Read the model definition and answer for the solid it produces. Units are mm, in the model's axes. A direction names the side the tool comes from. Give positions to 0.01 mm unless a question says otherwise; leave off trailing zeros. Order: outer loops, then holes, each group sorted by start corner. A loop starts at its lowest first (then second) coordinate and runs counter-clockwise, first axis right, second up. Notation, with made-up numbers: (-16.5, -30) -> (38.5, -30) arc R21 ccw to (38.5, -18) -> close; hole circle Ø10 at (9.5, 49.25). An arc over 180 degrees is marked (long way). Use one line per item in the form item = value.
```python
from build123d import *

# Parameters (mm, degrees)
SALIENTE_EXTRUIR1_DEPTH = 2
SALIENTE_EXTRUIR2_DEPTH = 24
CROQUIS4_W              = 26.838471133
CROQUIS4_H              = 14
CORTAR_EXTRUIR1_DEPTH   = 70.1
SALIENTE_EXTRUIR3_DEPTH = 2
SALIENTE_EXTRUIR4_DEPTH = 2
CROQUIS7_W              = 41.5
CROQUIS7_H              = 2
SALIENTE_EXTRUIR5_DEPTH = 8
SALIENTE_EXTRUIR6_DEPTH = 6


with BuildPart() as part:
    # Croquis1 → Saliente-Extruir1 (new body)
    with BuildSketch(Plane.XY):
        Polygon((-48.939551095, 26.503456625), (-8.439551095, 26.503456625), (-8.439551095, 6.503456625), (-8.439551095, 5.503456625), (-48.939551095, 5.503456625), (-49.939551095, 5.503456625), (-49.939551095, 26.503456625), align=None)
    extrude(amount=SALIENTE_EXTRUIR1_DEPTH)

    # Croquis3 → Saliente-Extruir2 (add)
    with BuildSketch(Plane.XY):
        Polygon((-48.939551095, 26.503456625), (-8.439551095, 26.503456625), (-8.439551095, 6.503456625), (-8.439551095, 5.503456625), (-48.939551095, 5.503456625), (-49.939551095, 5.503456625), (-49.939551095, 26.503456625), align=None)
        Polygon((-46.939551095, 7.503456625), (-47.939551095, 7.503456625), (-47.939551095, 24.503456625), (-46.939551095, 24.503456625), (-10.439551095, 24.503456625), (-10.439551095, 8.503456625), (-10.439551095, 7.503456625), align=None, mode=Mode.SUBTRACT)
    extrude(amount=SALIENTE_EXTRUIR2_DEPTH)

    # Croquis4 → Cortar-Extruir1 (cut)
    with BuildSketch(Plane(origin=(0, 0, 0), x_dir=(0, 0, -1), z_dir=(1, 0, 0))):
        with Locations((-15.419235567, 16.503456625)):
            Rectangle(CROQUIS4_W, CROQUIS4_H)
    extrude(amount=-CORTAR_EXTRUIR1_DEPTH, mode=Mode.SUBTRACT)

    # Croquis5 → Saliente-Extruir3 (add)
    with BuildSketch(Plane(origin=(0, 26.503456625, 0), x_dir=(1, 0, 0), z_dir=(0, 1, 0))):
        Polygon((-49.939551095, -20.607192887), (-8.439551095, -20.607192887), (-8.439551095, -24), (-8.439551095, -36.1), (-48.939551095, -36.1), (-49.939551095, -36.1), align=None)
    extrude(amount=-SALIENTE_EXTRUIR3_DEPTH)

    # Croquis6 → Saliente-Extruir4 (add)
    with BuildSketch(Plane.XY.offset(36.1)):
        Polygon((-8.439551095, 24.503456625), (-8.439551095, 33.503456625), (-48.939551095, 33.503456625), (-49.939551095, 33.503456625), (-49.939551095, 24.503456625), align=None)
    extrude(amount=-SALIENTE_EXTRUIR4_DEPTH)

    # Croquis7 → Saliente-Extruir5 (add)
    with BuildSketch(Plane.XY.offset(36.1)):
        with Locations((-29.189551095, 32.503456625)):
            Rectangle(CROQUIS7_W, CROQUIS7_H)
    extrude(amount=-SALIENTE_EXTRUIR5_DEPTH)

    # Croquis8 → Saliente-Extruir6 (add)
    with BuildSketch(Plane.XY.offset(36.1)):
        Polygon((-49.939551095, 29.503456625), (-49.939551095, 26.503456625), (-49.715027183, 26.503456625), (-8.439551095, 26.503456625), (-8.439551095, 29.503456625), (-49.715027183, 29.503456625), align=None)
    extrude(amount=-SALIENTE_EXTRUIR6_DEPTH)


solid = part.part
```
Item 1: The part is cut by section C-C on y = 27.25. Give the vertices of the cut face in (x, z).
Checks:
outline = (-49.94, 30.1) -> (-8.44, 30.1) -> (-8.44, 36.1) -> (-49.94, 36.1) -> close
Item 2: Which of the six approach directions +Z, -Z, +X, -X, +Y, -Y give full straight-line access (tool end or side, diameter ignored) to faces 1 (the flat face through (-10.44, 24, 13)), 2 (the flat face through (-49, 24, 24)), 3 (the flat face through (-49, 9.503, 13)), 4 (the flat face through (-29, 33.503, 32)), 5 (the flat face through (-29, 28, 30.1))?
Checks:
face_1 = +Z
face_2 = +Z, +X, -X, -Y
face_3 = +Z, +X, -X
face_4 = +Z, -Z, +X, -X, +Y
face_5 = -Z, +X, -X
Item 3: Determine the mould class of faces 6 (the flat face through (-29, 29, 36.1)), 7 (the flat face through (-29, 24.503, 19)), 8 (the flat face through (-29, 5.503, 12)) for opening direction Y: +Y half, -Y half, draft (parallel to the pull), parting line (faces both ways), or undercut.
Checks:
face_6 = draft
face_7 = undercut
face_8 = -Y half
Item 4: The part is cut by section A-A on z = 4.5. Give the vertices of the cut face in (x, y).
Checks:
outline = (-49.94, 5.5) -> (-8.44, 5.5) -> (-8.44, 9.5) -> (-10.44, 9.5) -> (-10.44, 7.5) -> (-47.94, 7.5) -> (-47.94, 9.5) -> (-49.94, 9.5) -> close; (-49.94, 23.5) -> (-47.94, 23.5) -> (-47.94, 24.5) -> (-10.44, 24.5) -> (-10.44, 23.5) -> (-8.44, 23.5) -> (-8.44, 26.5) -> (-49.94, 26.5) -> close
Item 5: The part is cut by section B-B on x = -11.5. Give the vertices of the cut face in (y, z).
Checks:
outline = (5.5, 0) -> (26.5, 0) -> (26.5, 30.1) -> (29.5, 30.1) -> (29.5, 34.1) -> (31.5, 34.1) -> (31.5, 28.1) -> (33.5, 28.1) -> (33.5, 36.1) -> (24.5, 36.1) -> (24.5, 2) -> (7.5, 2) -> (7.5, 24) -> (5.5, 24) -> close
Item 6: The part is cut by section D-D on z = 26.5. Give the vertices of the cut face in (x, y).
Checks:
outline = (-49.94, 24.5) -> (-8.44, 24.5) -> (-8.44, 26.5) -> (-49.94, 26.5) -> close
Item 7: Given pin 1 Ø2 at (x, y) = (-40, 9.5) entering from +Z; pin 2 Ø3 at (x, z) = (-37, 31) entering from -Y; pin 3 Ø1.6 at (x, z) = (-9, 14) entering from +Y, each flat-ended and moving along its own axis, determine where each tip first touches the part or whether it passes through.
Checks:
pin_1 = 2
pin_2 = 24.5
pin_3 = 26.5
Item 8: Straight lines are drawn through the part: L1, parallel to Y at x = -46, z = 32; L2, parallel to Y at x = -25, z = 12; L3, parallel to Z at x = -20.5, y = 17. For each, find the intervals that lie inside material, in ascending order. Write a range as from..to.
Checks:
L1 = 24.5..29.5, 31.5..33.5
L2 = 5.5..7.5, 24.5..26.5
L3 = 0..2
